Source: three-view drawing plus pictorial views. Frame: mm from the lowest corner of the part. A direction names the side the tool comes from. Give positions to 0.01 mm unless a question says otherwise; leave off trailing zeros. Write each loop counter-clockwise with the first axis right and the second up, starting at its lowest first coordinate (ties: lowest second). Pieces come first, ordered by that corner, then holes.
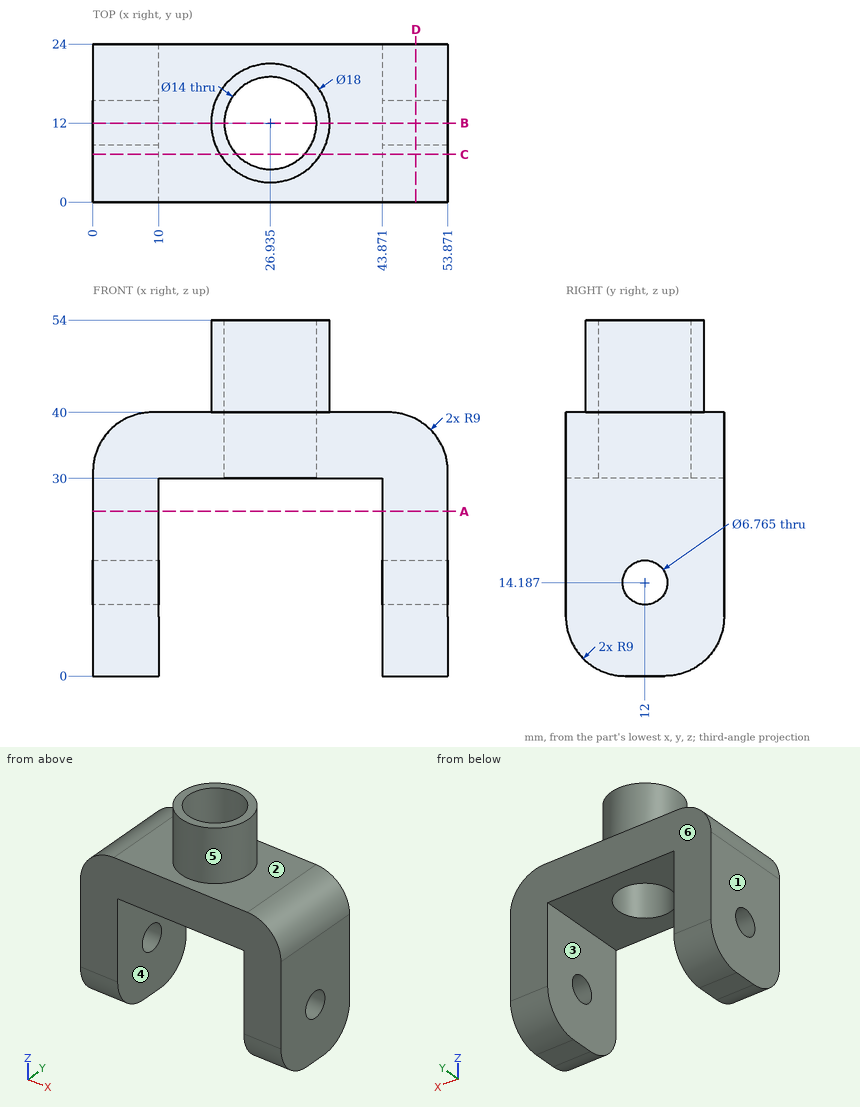
Q1. Pin query (flat end, axial travel): P1, Ø3, axis at x = 6, y = 16, coming from the +Z side; P2, Ø8, axis at x = 33, y = 21, coming from the -Z side; P3, Ø3, axis at y = 12, z = 40, coming from the -X side (1 decimal); P4, Ø12.5, axis at x = 26.94, y = 12, coming from the -Z side. Return the tip coordinate at first contact, or that it passes through.
Filled sheet:
P1: stops at z = 39.87
P2: stops at z = 30
P3: stops at x = 4
P4: passes through
Q2. Access query for the marked faces 1, 2 and 3. Directions: +Z, -Z, +X, -X, +Y, -Y. A direction counts if a zero-diameter tool reaches every point of the face in a straight line with its end or side. Return the directions, or none.
Filled sheet:
face 1: +Z, -Z, -X, +Y, -Y
face 2: +Z
face 3: -Z, +Y, -Y
Q3. Section B-B on y = 12. Output: boundary loops of the cut face in (x, z) (1 decimal).
Filled sheet:
outline: (0, 0) - (10, 0) - (10, 10.8) - (0, 10.8) - close; (0, 17.6) - (10, 17.6) - (10, 30) - (19.9, 30) - (19.9, 54) - (17.9, 54) - (17.9, 40) - (9, 40) arc R9 ccw to (0, 31) - close; (33.9, 30) - (43.9, 30) - (43.9, 17.6) - (53.9, 17.6) - (53.9, 31) arc R9 ccw to (44.9, 40) - (35.9, 40) - (35.9, 54) - (33.9, 54) - close; (43.9, 0) - (53.9, 0) - (53.9, 10.8) - (43.9, 10.8) - close
Q4. Section A-A on z = 25. Output: boundary loops of the cut face in (x, y), plus the area to 3 significant figures.
Filled sheet:
outline: (0, 0) - (10, 0) - (10, 24) - (0, 24) - close; (43.87, 0) - (53.87, 0) - (53.87, 24) - (43.87, 24) - close
area: 480 mm2
Q5. Section C-C on y = 7.25. Output: boundary loops of the cut face in (x, z).
Filled sheet:
outline: (0, 0.17) - (10, 0.17) - (10, 30) - (21.79, 30) - (21.79, 54) - (19.29, 54) - (19.29, 40) - (9, 40) arc R9 ccw to (0, 31) - close; (32.08, 30) - (43.87, 30) - (43.87, 0.17) - (53.87, 0.17) - (53.87, 31) arc R9 ccw to (44.87, 40) - (34.58, 40) - (34.58, 54) - (32.08, 54) - close
Q6. Section D-D on x = 49. Output: boundary loops of the cut face in (y, z) (1 decimal).
Filled sheet:
outline: (0, 9) arc R9 ccw to (9, 0) - (15, 0) arc R9 ccw to (24, 9) - (24, 39) - (0, 39) - close; hole circle Ø6.8 at (12, 14.2)
Q7. Ray query, line 1 along X through (y, z) = (20.5, 13.5); line 2 along Z through (x, y) = (19, 18.25); line 3 along X through (y, z) = (12.5, 42). Return the intervals inside material, ascending.
Filled sheet:
line 1: x = 0 to 10, 43.87 to 53.87
line 2: z = 30 to 40
line 3: x = 17.95 to 19.95, 33.92 to 35.92
Q8. Pull-direction query (X, two-part tool) for the marked faces 4, 5 and 6; classes: released by +X, released by -X, zero draft, split by the parting line, or undercut.
Filled sheet:
face 4: undercut
face 5: split by the parting line
face 6: zero draft
